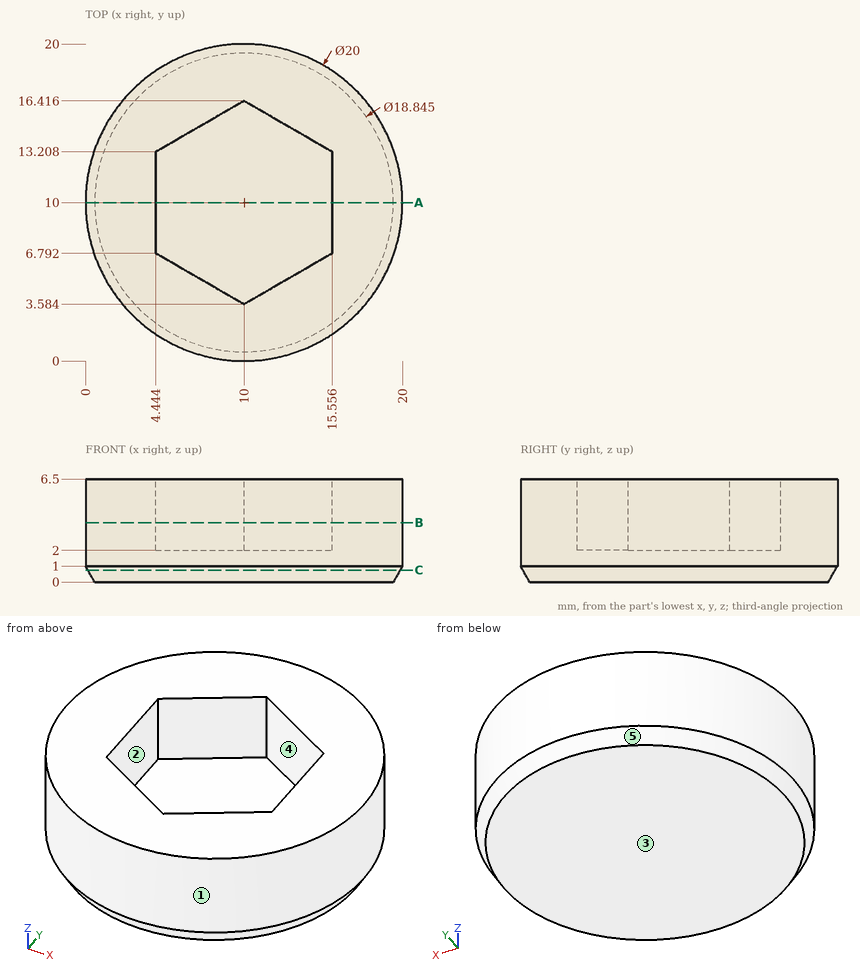
Input: dimensioned drawing with shaded views. Units: mm. Origin: part minimum x, y, z. A direction names the side the tool comes from. Round coordinates to 2 decimals unless told otherwise and drop trailing zeros. Order: outer loops, then holes, each group sorted by start corner. A loop starts at its lowest first (then second) coordinate and runs counter-clockwise, first axis right, second up.
1. Set-up query: the marked faces 4 and 5. Return all of +Z, -Z, +X, -X, +Y, -Y with unobstructed straight access to the full face (end or side cutting, diameter ignored); none if empty.
The answers:
face 4: +Z
face 5: -Z
2. Cut plane B-B, the plane z = 3.75. Output: boundary loops of the cut face in (x, y).
The answers:
outline: circle Ø20 at (10, 10); hole (4.44, 6.79) - (10, 3.58) - (15.56, 6.79) - (15.56, 13.21) - (10, 16.42) - (4.44, 13.21) - close
3. Cut plane A-A, the plane y = 10. Output: boundary loops of the cut face in (x, z).
The answers:
outline: (0, 1) - (0.58, 0) - (19.42, 0) - (20, 1) - (20, 6.5) - (15.56, 6.5) - (15.56, 2) - (4.44, 2) - (4.44, 6.5) - (0, 6.5) - close
4. Cut plane C-C, the plane z = 0.75. Output: boundary loops of the cut face in (x, y), then the cut area to 3 significant figures.
The answers:
outline: circle Ø19.71 at (10, 10)
area: 305 mm2
5. Pin query (flat end, axial travel): P1, Ø5, axis at x = 14.5, y = 13, coming from the +Z side; P2, Ø3, axis at y = 14.5, z = 3, coming from the -X side; P3, Ø4, axis at x = 11, y = 9.5, coming from the +Z side. Return the tip coordinate at first contact, or that it passes through.
The answers:
P1: stops at z = 6.5
P2: stops at x = 0.46
P3: stops at z = 2
6. Material intervals for line 1 (Z direction, x = 14.5, y = 11); line 2 (Y direction, x = 5.25, z = 4); line 3 (X direction, y = 5.25, z = 5.75) (1 decimal), sorted ascending.
The answers:
line 1: z = 0 to 2
line 2: y = 1.2 to 6.33, 13.67 to 18.8
line 3: x = 1.2 to 7.1, 12.9 to 18.8
7. Mould query, pull axis Y, two halves, no side actions, for the marked faces 1, 2 and 3. Classes: released by +Y, released by -Y, zero draft, split by the parting line, or undercut.
The answers:
face 1: split by the parting line
face 2: undercut
face 3: zero draft
